Check sheet for the modelled part. Datum: model origin and axes. Units: mm. A direction names the side the tool comes from. Coordinates: 2 decimals unless noted, no trailing zeros. Order: outer loops, then holes, each group sorted by start corner. A loop starts at its lowest first (then second) coordinate and runs counter-clockwise, first axis right, second up.
1. Gauge pin test, flat ends, axial feed: pin 1 Ø14.5 at (x, z) = (14.5, 2.5) entering from +Y; pin 2 Ø4 at (x, y) = (-63.5, 14) entering from -Z; pin 3 Ø8 at (y, z) = (6.5, 17) entering from -X. Record the tip position at first contact, or that the pin passes through.
2. Draft check along X on faces 1 (the cylindrical face through (25, 8, 0)), 2 (the flat face through (45, 6, 0)), 3 (the cylindrical face through (-29.014, 27.608, 0.661)). Enter one of: released by +X, released by -X, zero draft, split by the parting line, or undercut.
3. Cross-section at D-D (z = -12.5). Enter the section's corners in (x, y).
4. Set-up check for faces 4 (the flat face through (-65, 28, -3)), 5 (the flat face through (5, 18, 0)), 6 (the flat face through (0, 0, 0)): record each of +Z, -Z, +X, -X, +Y, -Y from which the full face is reachable in a straight line by a thin tool's end or side.
5. Cross-section at A-A (z = 0). Enter the section's corners in (x, y), then the cut area to 3 significant figures.
6. Cross-section at C-C (x = 32). Enter the section's corners in (y, z).
7. Thickness scan on line 1 (Z direction, x = -45, y = 20.5); line 2 (X direction, y = 18.5, z = -12.5); line 3 (Z direction, x = -50, y = 25). Record the ranges inside material, lowest first.
8. Cross-section at B-B (y = 4.5). Enter the section's corners in (x, z).
```python
from build123d import *

# Parameters (mm, degrees)
SKETCH1_W                = 90
SKETCH1_H                = 48
BOSS_EXTRUDE1_DEPTH      = 24
SKETCH8_R                = 16
CUT_EXTRUDE1_DEPTH       = 40
BOSS_EXTRUDE2_DEPTH      = 32
BOSS_EXTRUDE2_DEPTH_BACK = 24
SKETCH9_R                = 24
SKETCH9_R_2              = 16
CUT_EXTRUDE2_DEPTH       = 32
CUT_EXTRUDE2_DEPTH_BACK  = 24
SKETCH10_R               = 16
SKETCH11_W               = 22
SKETCH11_H               = 6
CUT_EXTRUDE3_DEPTH       = 93.048900048


with BuildPart() as part:
    # Sketch1 → Boss-Extrude1 (new body)
    with BuildSketch(Plane(origin=(0, 0, 0), x_dir=(1, 0, 0), z_dir=(0, 1, 0))):
        Rectangle(SKETCH1_W, SKETCH1_H)
    extrude(amount=BOSS_EXTRUDE1_DEPTH)

    # Sketch8 → Cut-Extrude1 (cut)
    with BuildSketch(Plane(origin=(45, 0, 0), x_dir=(0, 0, -1), z_dir=(1, 0, 0))):
        with Locations((0, 24)):
            Circle(SKETCH8_R)
    extrude(amount=-CUT_EXTRUDE1_DEPTH, mode=Mode.SUBTRACT)

    # Sketch9 → Boss-Extrude2 (add, two sides: drawn at the far end of the back side and taken through both)
    with BuildSketch(Plane(origin=(0, 24, 0), x_dir=(1, 0, 0), z_dir=(0, 1, 0)).offset(-BOSS_EXTRUDE2_DEPTH_BACK)):
        with Locations(Location((-45, 0, 0), (0, 0, 270))):
            Circle(SKETCH9_R)
        with Locations(Location((-45, 0, 0), (0, 0, 270))):
            Circle(SKETCH9_R_2, mode=Mode.SUBTRACT)
    extrude(amount=BOSS_EXTRUDE2_DEPTH + BOSS_EXTRUDE2_DEPTH_BACK)

    # Sketch10 → Cut-Extrude2 (cut, two sides: drawn at the far end of the back side and taken through both)
    with BuildSketch(Plane(origin=(0, 24, 0), x_dir=(1, 0, 0), z_dir=(0, 1, 0)).offset(-CUT_EXTRUDE2_DEPTH_BACK)):
        with Locations(Location((-45, 0, 0), (0, 0, 270))):
            Circle(SKETCH10_R)
    extrude(amount=CUT_EXTRUDE2_DEPTH + CUT_EXTRUDE2_DEPTH_BACK, mode=Mode.SUBTRACT)

    # Sketch11 → Cut-Extrude3 (cut, through all)
    with BuildSketch(Plane(origin=(0, 56, 0), x_dir=(1, 0, 0), z_dir=(0, 1, 0))):
        with Locations((-69, 0)):
            Rectangle(SKETCH11_W, SKETCH11_H)
    extrude(amount=-CUT_EXTRUDE3_DEPTH, mode=Mode.SUBTRACT)


solid = part.part
```
Data:
1. pin 1: stops at y = 11.31
1. pin 2: stops at z = -17.43
1. pin 3: stops at x = -65.17
2. face 1: zero draft
2. face 2: released by +X
2. face 3: undercut
3. outline: (-65.49, 0) - (-54.99, 0) - (-54.99, 56) - (-65.49, 56) - close; (-35.01, 0) - (45, 0) - (45, 14.01) - (5, 14.01) - (5, 24) - (-24.51, 24) - (-24.51, 56) - (-35.01, 56) - close
4. face 4: -X, +Y, -Y
4. face 5: +X, +Y
4. face 6: +Z, -Z, +X, -X, -Y
5. outline: (-29, 0) - (45, 0) - (45, 8) - (5, 8) - (5, 24) - (-21, 24) - (-21, 56) - (-29, 56) - close
5. area: 1,390 mm2
6. outline: (0, -24) - (24, -24) - (24, -16) arc R16 cw to (24, 16) - (24, 24) - (0, 24) - close
7. line 1: z = -24 to -16, 16 to 24
7. line 2: x = -65.49 to -54.99, -35.01 to 5
7. line 3: z = -23.47 to -15.2, 15.2 to 23.47
8. outline: (-68.81, -3) arc R24 ccw to (-45, -24) - (45, -24) - (45, 24) - (-45, 24) arc R24 ccw to (-68.81, 3) - (-60.72, 3) arc R16 cw (long way) to (-60.72, -3) - close
